Model file for the job. Use its own axes, mm. Give positions to 0.01 mm unless a question says otherwise; leave off trailing zeros. Loops run counter-clockwise (first coordinate to the right, second up) from the corner with the lowest first, then second, coordinate; pieces in that order, holes last. Notation, with made-up numbers: (61, -1) -> (104, -1) arc R14 ccw to (104, 18) -> close; hole circle Ø7 at (14.25, 31.5). An arc over 180 degrees is marked (long way). Use CSV: the item, a comma, the result in double quotes. Start each with the question number.
(1) Pull direction X, two halves, no side cores. Call faces 1 (the flat face through (13, -9, 24)), 2 (the flat face through (-7.33, 14.75, 13.15)): pulls with the +X half, pulls with the -X half, needs draft (parallel to the pull), parting line crosses it, or undercut.
(2) Cut at D-D on z = 12.5. State how many separate pieces and enclosed holes the cut face has, then the cut area to 3 significant figures.
(3) Flat gauge pins, fed straight in: pin 1 (2 mm diameter, centred on x = -28, y = -17.5, fed in from +Z); pin 2 (1 mm diameter, centred on x = 31.5, z = 9.5, fed in from -Y); pin 3 (5 mm diameter, centred on y = -28, z = 18, fed in from -X). Where does each tip first touch, or does it go through?
(4) Cut at B-B on y = -10. Write the cut outline in (x, z), then the cut area to 3 significant figures.
(5) Cut at A-A on x = 0. Write the cut outline in (y, z).
(6) Drill centre lines: probe 1 along Y at (x, z) = (0, 8.75); probe 2 along X at (y, z) = (-32.5, 14.75); probe 3 along X at (y, z) = (-23, 20.75). Where is each one in solid material? Low to high.
(7) Cut at C-C on x = -20.5. Write the cut outline in (y, z) (3 decimals).
from build123d import *

# Parameters (mm, degrees)
F0_R     = 43
F0_R_2   = 15
F1_DEPTH = 24
F3_DEPTH = 22


with BuildPart() as f1:
    # F0 (on Top) → F1 (new body)
    with BuildSketch(Plane.XY):
        Circle(F0_R)
        Circle(F0_R_2, mode=Mode.SUBTRACT)
    extrude(amount=F1_DEPTH)

    # F2 (on face) → F3 (cut)
    with BuildSketch(Plane.XY.offset(24)):
        with BuildLine():
            Line((-11.312369, 12.229999), (-26.267696, 30.978592))
            ThreePointArc((-26.267696, 30.978592), (-31.908319, 25.231136), (-36.256517, 18.453006))
            Line((-36.256517, 18.453006), (-14.650118, 8.044594))
            Line((-14.650118, 8.044594), (-11.312369, 12.229999))
        make_face()
        with BuildLine():
            Line((-4.885694, 15.927101), (-10.225269, 39.307873))
            ThreePointArc((-10.225269, 39.307873), (-17.801022, 36.576969), (-24.659534, 32.356697))
            Line((-24.659534, 32.356697), (-9.708882, 13.604377))
            Line((-9.708882, 13.604377), (-4.885694, 15.927101))
        make_face()
        with BuildLine():
            Line((2.508652, 16.469646), (7.842398, 39.851748))
            ThreePointArc((7.842398, 39.851748), (-0.168015, 40.678284), (-8.178428, 39.851748))
            Line((-8.178428, 39.851748), (-2.844682, 16.469646))
            Line((-2.844682, 16.469646), (2.508652, 16.469646))
        make_face()
        with BuildLine():
            Line((9.406129, 13.750175), (24.356781, 32.502495))
            ThreePointArc((24.356781, 32.502495), (17.49827, 36.722767), (9.922517, 39.453671))
            Line((9.922517, 39.453671), (4.582941, 16.072899))
            Line((4.582941, 16.072899), (9.406129, 13.750175))
        make_face()
        with BuildLine():
            Line((14.440607, 8.307313), (36.047006, 18.715725))
            ThreePointArc((36.047006, 18.715725), (31.698808, 25.493855), (26.058185, 31.24131))
            Line((26.058185, 31.24131), (11.102857, 12.492718))
            Line((11.102857, 12.492718), (14.440607, 8.307313))
        make_face()
        with BuildLine():
            Line((16.614945, 1.219086), (40.597679, 1.222076))
            ThreePointArc((40.597679, 1.222076), (39.621008, 9.215572), (37.03271, 16.841225))
            Line((37.03271, 16.841225), (15.423716, 6.438201))
            Line((15.423716, 6.438201), (16.614945, 1.219086))
        make_face()
        with BuildLine():
            Line((15.49849, -6.110596), (37.107484, -16.51362))
            ThreePointArc((37.107484, -16.51362), (39.695782, -8.887967), (40.672453, -0.894471))
            Line((40.672453, -0.894471), (16.689719, -0.891481))
            Line((16.689719, -0.891481), (15.49849, -6.110596))
        make_face()
        with BuildLine():
            Line((11.312369, -12.229999), (26.267696, -30.978592))
            ThreePointArc((26.267696, -30.978592), (31.908319, -25.231136), (36.256517, -18.453006))
            Line((36.256517, -18.453006), (14.650118, -8.044594))
            Line((14.650118, -8.044594), (11.312369, -12.229999))
        make_face()
        with BuildLine():
            Line((4.885694, -15.927101), (10.225269, -39.307873))
            ThreePointArc((10.225269, -39.307873), (17.801022, -36.576969), (24.659534, -32.356697))
            Line((24.659534, -32.356697), (9.708882, -13.604377))
            Line((9.708882, -13.604377), (4.885694, -15.927101))
        make_face()
        with BuildLine():
            Line((-2.508652, -16.469646), (-7.842398, -39.851748))
            ThreePointArc((-7.842398, -39.851748), (0.168015, -40.678284), (8.178428, -39.851748))
            Line((8.178428, -39.851748), (2.844682, -16.469646))
            Line((2.844682, -16.469646), (-2.508652, -16.469646))
        make_face()
        with BuildLine():
            Line((-9.406129, -13.750175), (-24.356781, -32.502495))
            ThreePointArc((-24.356781, -32.502495), (-17.49827, -36.722767), (-9.922517, -39.453671))
            Line((-9.922517, -39.453671), (-4.582941, -16.072899))
            Line((-4.582941, -16.072899), (-9.406129, -13.750175))
        make_face()
        with BuildLine():
            Line((-14.440607, -8.307313), (-36.047006, -18.715725))
            ThreePointArc((-36.047006, -18.715725), (-31.698808, -25.493855), (-26.058185, -31.24131))
            Line((-26.058185, -31.24131), (-11.102857, -12.492718))
            Line((-11.102857, -12.492718), (-14.440607, -8.307313))
        make_face()
        with BuildLine():
            Line((-16.614945, -1.219086), (-40.597679, -1.222076))
            ThreePointArc((-40.597679, -1.222076), (-39.621008, -9.215572), (-37.03271, -16.841225))
            Line((-37.03271, -16.841225), (-15.423716, -6.438201))
            Line((-15.423716, -6.438201), (-16.614945, -1.219086))
        make_face()
        with BuildLine():
            Line((-15.49849, 6.110596), (-37.107484, 16.51362))
            ThreePointArc((-37.107484, 16.51362), (-39.695782, 8.887967), (-40.672453, 0.894471))
            Line((-40.672453, 0.894471), (-16.689719, 0.891481))
            Line((-16.689719, 0.891481), (-15.49849, 6.110596))
        make_face()
    extrude(amount=-F3_DEPTH, mode=Mode.SUBTRACT)


solid = f1.part
Check result:
1,face 1,"needs draft"
1,face 2,"undercut"
2,separate pieces,"1"
2,enclosed holes,"15"
2,area,"1,480 mm²"
3,pin 1,"z = 2"
3,pin 2,"y = -29.8"
3,pin 3,"x = -34.62"
4,outline,"(-41.82, 0) -> (-11.18, 0) -> (-11.18, 24) -> (-13.09, 24) -> (-13.09, 2) -> (-17.95, 2) -> (-17.95, 24) -> (-22.82, 24) -> (-22.82, 2) -> (-39.43, 2) -> (-39.43, 24) -> (-41.82, 24) -> close; (11.18, 0) -> (41.82, 0) -> (41.82, 24) -> (39.42, 24) -> (39.42, 2) -> (23.58, 2) -> (23.58, 24) -> (18.71, 24) -> (18.71, 2) -> (13.09, 2) -> (13.09, 24) -> (11.18, 24) -> close"
4,area,"526 mm²"
5,outline,"(-43, 0) -> (-15, 0) -> (-15, 24) -> (-16.47, 24) -> (-16.47, 2) -> (-40.68, 2) -> (-40.68, 24) -> (-43, 24) -> close; (15, 0) -> (43, 0) -> (43, 24) -> (40.68, 24) -> (40.68, 2) -> (16.47, 2) -> (16.47, 24) -> (15, 24) -> close"
6,probe 1,"-43 to -40.68, -16.47 to -15, 15 to 16.47, 40.68 to 43"
6,probe 2,"-28.16 to -24.35, -8.33 to -6.17, 6.5 to 8.67, 24.47 to 28.16"
6,probe 3,"-36.33 to -33.53, -19.48 to -16.78, -6.16 to -4, 4.33 to 6.5, 17.2 to 19.9, 33.56 to 36.33"
7,outline,"(-37.799, 0) -> (37.799, 0) -> (37.799, 24) -> (35.145, 24) -> (35.145, 2) -> (27.139, 2) -> (27.139, 24) -> (23.748, 24) -> (23.748, 2) -> (10.863, 2) -> (10.863, 24) -> (8.518, 24) -> (8.518, 2) -> (0.892, 2) -> (0.892, 24) -> (-1.22, 24) -> (-1.22, 2) -> (-8.882, 2) -> (-8.882, 24) -> (-11.226, 24) -> (-11.226, 2) -> (-24.273, 2) -> (-24.273, 24) -> (-27.665, 24) -> (-27.665, 2) -> (-35.113, 2) -> (-35.113, 24) -> (-37.799, 24) -> close"
